For this review, take the finished solid that the model builds, in its own axes (mm). Face numbers are marked on the shaded views. A direction names the side the tool comes from. Coordinates: 2 decimals unless noted, no trailing zeros. Order: outer loops, then holes, each group sorted by start corner. A loop starts at its lowest first (then second) coordinate and runs counter-clockwise, first axis right, second up. Notation, with made-up numbers: (-2, -26) -> (22, -26) arc R8 cw to (22, -17) -> close; hole circle Ø3 at (-19.75, -17). An arc over 180 degrees is marked (long way). Answer as a JSON object with one key per item and string values. Group by question number.
1) Machinability: for the marked faces 1, 2, 3 and 4, which of the approach directions +Z, -Z, +X, -X, +Y, -Y give a long, thin tool a straight path to every point of the face, cutting with its end or side? Answer none if there is none.
2) For pin 1 (0.5 mm diameter, centred on y = 11, z = 0.5, fed in from -X); pin 2 (1.1 mm diameter, centred on y = 10.5, z = 0.5, fed in from +X); pin 3 (0.5 mm diameter, centred on x = 10.5, z = 0.5, fed in from +Y), all flat-tipped, find the tip position at first contact; note any pin that passes through.
3) Wall thickness on L1, parallel to Y at x = 8, z = 1.65; L2, parallel to Y at x = 2, z = 0.35; L3, parallel to Z at x = 1.75, y = 8.5: over which ranges is each line inside the solid? List them lowest first.
4) Add section D-D, the plane y = 2.25. Write out the cut boundary in (x, z), then the cut area to 3 significant figures.
5) Draft analysis for pull direction Y (two halves, no side actions). For the marked faces 5, 6 and 7, state which applies: +Y half, -Y half, draft (parallel to the pull), parting line (faces both ways), or undercut.
6) Add section C-C, the plane y = 11.5. Write out the cut boundary in (x, z), then the cut area to 3 significant figures.
7) Add section B-B, the plane z = 1.6. Write out the cut boundary in (x, y).
8) Add section A-A, the plane x = 5.75. Write out the cut boundary in (y, z), then the cut area to 3 significant figures.
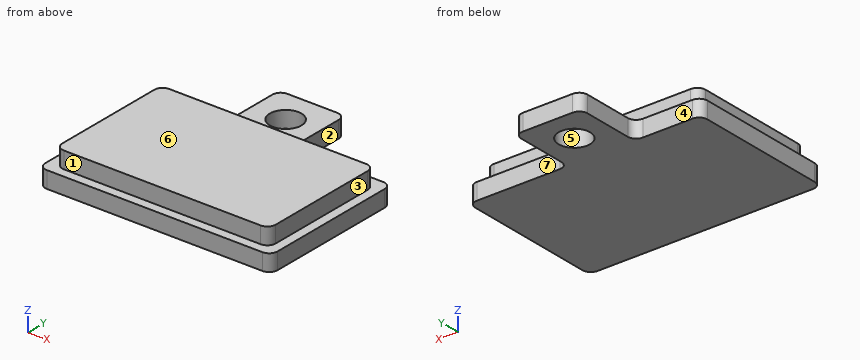
Autodesk Inventor part; units mm, degrees
ref_plane "YZ Plane" through (0, 0, 0) normal (1, 0, 0) x (0, 1, 0)
ref_plane "XZ Plane" through (0, 0, 0) normal (0, 1, 0) x (-1, 0, 0)
ref_plane "XY Plane" through (0, 0, 0) normal (0, 0, 1) x (1, 0, 0)
sketch "Sketch1" plane through (0, 0, 0) normal (0, 0, 1) x (1, 0, 0)
  line L0 (0, 0) -> (14, 0)
  line L1 (14, 0) -> (14, 9)
  line L2 (14, 9) -> (0, 9)
  line L3 (0, 9) -> (0, 0)
  dimension "d0" = 14
  dimension "d1" = 9
extrude "Extrusion1" add sketch "Sketch1" along normal blind 2
sketch "Sketch2" plane through (0, 0, 2) normal (0, 0, 1) x (1, 0, 0)
  line L0 (0, 0) -> (0, 9)
  line L1 (14, 0) -> (0, 0)
  line L2 (14, 9) -> (14, 0)
  line L3 (0, 9) -> (14, 9)
  line L4 (0.5635, 8.4365) -> (0.5635, 0.5635)
  line L5 (0.5635, 0.5635) -> (13.4365, 0.5635)
  line L6 (13.4365, 0.5635) -> (13.4365, 8.4365)
  line L7 (13.4365, 8.4365) -> (0.5635, 8.4365)
  dimension "d4" = 0.5635
extrude "Extrusion2" cut sketch "Sketch2" against normal blind 1
sketch "Sketch3" plane through (0, 9, 0) normal (0, 1, 0) x (1, 0, 0)
  line L0 (0, -1) -> (14, -1)
  line L1 (14, 0) -> (0, 0)
  line L2 (0, 0) -> (0, -1)
  line L3 (4, 0) -> (8, 0)
  line L4 (8, 0) -> (8, -1)
  line L5 (8, -1) -> (4, -1)
  line L6 (4, -1) -> (4, 0)
  dimension "d7" = 4
  dimension "d8" = 4
extrude "Extrusion3" add sketch "Sketch3" along normal blind 4 contours L6 L1 L4 L0
sketch "Sketch4" plane through (0, 0, 1) normal (0, 0, 1) x (1, 0, 0)
  line L0 (8, 13) -> (4, 13)
  line L1 (4, 9) -> (4, 13)
  line L2 (0, 0) -> (0, 9)
  line L3 (4, 11) -> (8.8648, 11) construction
  line L4 (6, 13) -> (6, 6.8956) construction
  point P0 (6.0394, 10.9642)
hole "Hole1" at (6.0394, 10.9642, 1) direction (0, 0, -1) diameter 1.905 end through all
fillet "Fillet1" radius 0.5 12 edges at (0.5635, 0.5635, 1.5) (0, 0, 0.5) (0.5635, 8.4365, 1.5) (0, 9, 0.5) (13.4365, 0.5635, 1.5) (14, 0, 0.5) (13.4365, 8.4365, 1.5) (14, 9, 0.5) (8, 9, 0.5) (4, 9, 0.5) (4, 13, 0.5) (8, 13, 0.5)
properties part number "lid"
Output values:
{
 "1": {"face 1": "+Z, +X, -X, -Y", "face 2": "+Z, -Z, +X, +Y", "face 3": "+Z, +X, +Y, -Y", "face 4": "+Z, -Z, -X, +Y"},
 "2": {"pin 1": "stops at x = 4", "pin 2": "stops at x = 8", "pin 3": "stops at y = 9"},
 "3": {"L1": "y = 0.56 to 8.44", "L2": "y = 0 to 9", "L3": "z = 0 to 1"},
 "4": {"outline": "(0, 0) -> (14, 0) -> (14, 1) -> (13.44, 1) -> (13.44, 2) -> (0.56, 2) -> (0.56, 1) -> (0, 1) -> close", "area": "26.9 mm²"},
 "5": {"face 5": "undercut", "face 6": "draft", "face 7": "+Y half"},
 "6": {"outline": "(4, 0) -> (5.25, 0) -> (5.25, 1) -> (4, 1) -> close; (6.83, 0) -> (8, 0) -> (8, 1) -> (6.83, 1) -> close", "area": "2.42 mm²"},
 "7": {"outline": "(0.56, 1.06) arc R0.5 ccw to (1.06, 0.56) -> (12.94, 0.56) arc R0.5 ccw to (13.44, 1.06) -> (13.44, 7.94) arc R0.5 ccw to (12.94, 8.44) -> (1.06, 8.44) arc R0.5 ccw to (0.56, 7.94) -> close"},
 "8": {"outline": "(0, 0) -> (10.06, 0) -> (10.06, 1) -> (8.44, 1) -> (8.44, 2) -> (0.56, 2) -> (0.56, 1) -> (0, 1) -> close; (11.87, 0) -> (13, 0) -> (13, 1) -> (11.87, 1) -> close", "area": "19.1 mm²"}
}
